Geometry: final body of the model. Coordinates: model frame, mm. Face numbers are marked on the shaded views. A direction names the side the tool comes from. Round coordinates to 2 decimals unless told otherwise and drop trailing zeros. Order: outer loops, then holes, each group sorted by start corner. A loop starts at its lowest first (then second) coordinate and runs counter-clockwise, first axis right, second up. Notation, with made-up numbers: M 25.5,-6.5 L 60.5,-6.5 A15 ccw 60.5,6.5 Z; hole C -5,25.25 d10. An arc over 180 degrees is marked long. Return JSON: item names as keys, results as strings. Group by question number.
Q1. Ray query, probe 1 along Y at (x, z) = (17.5, 18); probe 2 along Y at (x, z) = (31, 26); probe 3 along X at (y, z) = (-31, 17). Return the intervals inside material, ascending.
Q2. Access query for the marked faces 1, 2 and 3. Directions: +Z, -Z, +X, -X, +Y, -Y. A direction counts if a zero-diameter tool reaches every point of the face in a straight line with its end or side. Return the directions, or none.
Q3. Cut plane C-C on z = 24. Count the separate pieces of the cut face and the enclosed holes in it, and give its area (3 significant figures).
Q4. Cut plane D-D on x = 12. Output: boundary loops of the cut face in (y, z) (3 decimals), and give its area (3 significant figures).
Q5. Cut plane A-A on z = 3.5. Output: boundary loops of the cut face in (x, y), and give its area (3 significant figures).
Q6. Contact query for flat-ended pins moving along their axis: pin 1 (10 mm diameter, centred on x = 15.5, z = 14, fed in from +Y); pin 2 (1 mm diameter, centred on x = 18.5, y = -15.5, fed in from -Z) (3 decimals); pin 3 (12 mm diameter, centred on x = 18, z = 18, fed in from -Y); pin 4 (1 mm diameter, centred on y = -21, z = 4.5, fed in from +X). Output: stop coordinate, or through.
Q7. Mould query, pull axis Y, two halves, no side actions, for the marked faces 4, 5 and 6. Classes: released by +Y, released by -Y, zero draft, split by the parting line, or undercut.
Q8. Cut plane B-B on x = 23. Output: boundary loops of the cut face in (y, z) (3 decimals), and give its area (3 significant figures).
```python
from build123d import *

# Parameters (mm, degrees)
F0_W      = 38.1
F0_H      = 38.1
F1_DEPTH  = 38.1
F6_DEPTH  = 38.1
F8_DEPTH  = 38.1
F9_W      = 25.4
F9_H      = 7.62
F10_DEPTH = 38.1


with BuildPart() as f1:
    # F0 (on Front) → F1 (new body)
    with BuildSketch(Plane.XZ):
        with Locations((19.05, 19.05)):
            Rectangle(F0_W, F0_H)
    extrude(amount=F1_DEPTH)

    # F5 (on offset) → F6 (cut)
    with BuildSketch(Plane.YZ.offset(38.1)):
        Polygon((-31.75, 0), (-38.1, 38.1), (-38.1, 0), align=None)
        Polygon((-19.05, 15.875), (-25.4, 0), (-12.7, 0), align=None)
        Polygon((0, 38.1), (-6.35, 0), (0, 0), align=None)
        Polygon((-6.35, 38.1), (-16.51, 38.1), (-16.51, 28.40746), (-10.16, 15.875), align=None)
        Polygon((-21.59, 38.1), (-31.75, 38.1), (-25.4, 15.875), (-20.336536, 28.53366), (-21.59, 28.575), align=None)
        Polygon((-16.51, 38.1), (-21.59, 38.1), (-21.59, 28.575), (-20.336536, 28.53366), (-20.32, 28.575), (-16.51, 28.40746), align=None)
    extrude(amount=-F6_DEPTH, mode=Mode.SUBTRACT)

    # F7 (on offset) → F8 (cut)
    with BuildSketch(Plane.XZ.offset(38.1)):
        Polygon((31.75, 38.1), (38.1, 0), (38.1, 38.1), align=None)
        Polygon((25.4, 38.1), (12.7, 38.1), (19.05, 22.225), align=None)
        Polygon((0, 38.1), (0, 0), (6.35, 38.1), align=None)
        Polygon((11.43, 22.225), (6.35, 0), (31.75, 0), (26.67, 22.225), (21.59, 9.525), (16.51, 9.525), align=None)
    extrude(amount=-F8_DEPTH, mode=Mode.SUBTRACT)

    # F9 (on offset) → F10 (cut)
    with BuildSketch(Plane.XY.offset(38.1)):
        with Locations((25.4, -11.43)):
            Rectangle(F9_W, F9_H)
        with Locations((12.7, -26.67)):
            Rectangle(F9_W, F9_H)
    extrude(amount=-F10_DEPTH, mode=Mode.SUBTRACT)


solid = f1.part
```
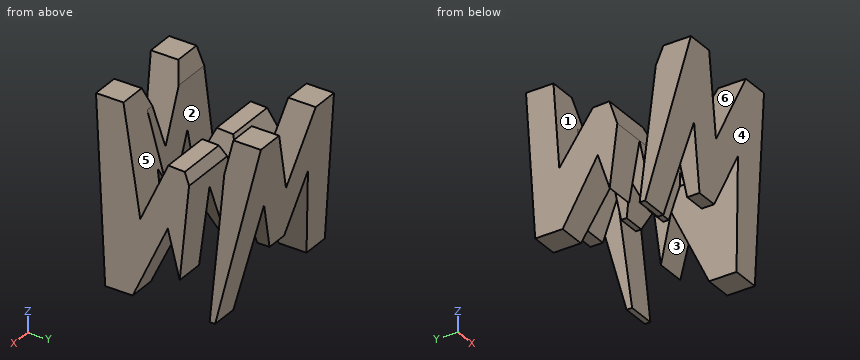
Result sheet:
{
 "1": {"probe 1": "y = -34.75 to -30.48, -22.86 to -15.24, -7.62 to -3.35", "probe 2": "y = -36.08 to -28.29, -21.35 to -15.29, -7.62 to -2.02", "probe 3": "x = 2.83 to 10.24, 13.52 to 24.58, 27.86 to 35.27"},
 "2": {"face 1": "+Z, +X, -X", "face 2": "+Z, -Z, -X", "face 3": "-Z, +X, -X"},
 "3": {"separate pieces": "6", "enclosed holes": "0", "area": "543 mm²"},
 "4": {"outline": "M -38.1,38.1 L -35.217,20.8 L -30.48,20.8 L -30.48,33.655 L -31.75,38.1 Z; M -22.86,20.8 L -12.655,20.8 L -16.51,28.407 L -20.32,28.575 L -22.86,22.225 Z; M -9.316,20.8 L -2.883,20.8 L 0,38.1 L -6.35,38.1 Z", "area": "270 mm²"},
 "5": {"outline": "M 0.58,-32.33 L 7.15,-32.33 L 7.15,-30.48 L 0.58,-30.48 Z; M 0.58,-14.1 L 7.15,-14.1 L 7.15,-5.77 L 0.58,-5.77 Z; M 30.95,-32.33 L 37.52,-32.33 L 37.52,-24 L 30.95,-24 Z; M 30.95,-7.62 L 37.52,-7.62 L 37.52,-5.77 L 30.95,-5.77 Z", "area": "134 mm²"},
 "6": {"pin 1": "stops at y = -3.18", "pin 2": "stops at z = 9.525", "pin 3": "stops at y = -35.75", "pin 4": "passes through"},
 "7": {"face 4": "released by -Y", "face 5": "undercut", "face 6": "zero draft"},
 "8": {"outline": "M -37.1,32.1 L -33.925,13.05 L -30.48,13.05 L -30.48,32.1 Z; M -22.86,13.05 L -20.18,13.05 L -19.05,15.875 L -17.92,13.05 L -15.24,13.05 L -15.24,25.901 L -16.51,28.407 L -20.32,28.575 L -22.86,22.225 Z; M -7.62,13.05 L -4.175,13.05 L -1,32.1 L -7.379,32.1 L -7.62,30.692 Z", "area": "296 mm²"}
}
